```python
from build123d import *

# Parameters (mm, degrees)
F0_R     = 35
F1_DEPTH = 25
F2_R     = 50
F2_R_2   = 35
F3_DEPTH = 25


# Not quite as in the source:
# - a pattern or mirror of a feature is missing from the dataset's text; its kind, count and spacing are read off the source's solid


with BuildPart() as f1:
    # F0 (on Front) → F1 (new body, symmetric)
    with BuildSketch(Plane.XZ):
        with BuildLine():
            Line((100, 70), (-100, 70))
            ThreePointArc((-100, 70), (-170, 0), (-100, -70))
            Line((-100, -70), (100, -70))
            ThreePointArc((100, -70), (170, 0), (100, 70))
        make_face()
        with Locations((-100, 0)):
            Circle(F0_R, mode=Mode.SUBTRACT)
        with Locations((100, 0)):
            Circle(F0_R, mode=Mode.SUBTRACT)
    extrude(amount=F1_DEPTH, both=True)

    # F2 (on face) → F3 (join)
    with BuildSketch(Plane.XZ.offset(25)):
        with Locations((100, 0)):
            Circle(F2_R)
        with Locations((100, 0)):
            Circle(F2_R_2, mode=Mode.SUBTRACT)
    f3 = extrude(amount=F3_DEPTH)

    # F3_copies: F3 across plane
    add(f3.mirror(Plane.ZX))


solid = f1.part
```
Check sheet for the modelled part. Datum: model origin and axes. Units: mm. A direction names the side the tool comes from. Coordinates: 2 decimals unless noted, no trailing zeros. Write each loop counter-clockwise with the first axis right and the second up, starting at its lowest first coordinate (ties: lowest second). Pieces come first, ordered by that corner, then holes. Notation, with made-up numbers: (-27.75, 6.25) - (18.25, 6.25) arc R31 cw to (18.25, 35.25) - close; hole circle Ø3 at (66, 6.25). An arc over 180 degrees is marked (long way). One line per question, with ' | ' between items.
Item 1: Sectioned sample at B-B on y = -16.5. Record the boundary of the cut face in (x, z), plus the area to 3 significant figures.
Determined:
outline: (-100, -70) - (100, -70) arc R70 ccw to (100, 70) - (-100, 70) arc R70 ccw to start; hole circle Ø70 at (-100, 0); hole circle Ø70 at (100, 0) | area: 35,700 mm2
Item 2: Sectioned sample at A-A on z = 0. Record the boundary of the cut face in (x, y), plus the area to 3 significant figures.
Determined:
outline: (-170, -25) - (-135, -25) - (-135, 25) - (-170, 25) - close; (-65, -25) - (50, -25) - (50, -50) - (65, -50) - (65, 50) - (50, 50) - (50, 25) - (-65, 25) - close; (135, -50) - (150, -50) - (150, -25) - (170, -25) - (170, 25) - (150, 25) - (150, 50) - (135, 50) - close | area: 11,500 mm2
Item 3: Sectioned sample at C-C on y = -36.5. Record the boundary of the cut face in (x, z), plus the area to 3 significant figures.
Determined:
outline: circle Ø100 at (100, 0); hole circle Ø70 at (100, 0) | area: 4,010 mm2
Item 4: Thickness scan on line 1 (Z direction, x = -100, y = 6); line 2 (X direction, y = -3, z = 21); line 3 (Z direction, x = 100, y = -28.5). Record the ranges inside material, lowest first. Write a range as [from, to].
Determined:
line 1: z = [-70, -35], [35, 70] | line 2: x = [-166.78, -128], [-72, 72], [128, 166.78] | line 3: z = [-50, -35], [35, 50]
Item 5: Sectioned sample at D-D on z = -54. Record the boundary of the cut face in (x, y).
Determined:
outline: (-144.54, -25) - (144.54, -25) - (144.54, 25) - (-144.54, 25) - close
Item 6: Mould release check, pull along Z, two halves, no side actions. Record for faces 1 (the face through (169.983, -0.35, -1.539)), 2 (the face through (1, 0, 70)), 3 (the face through (132.33, -0.7, -13.41)): pulls with the +Z half, pulls with the -Z half, needs draft (parallel to the pull), parting line crosses it, or undercut.
Determined:
face 1: parting line crosses it | face 2: pulls with the +Z half | face 3: undercut
Item 7: Gauge pin test, flat ends, axial feed: P1, Ø1, axis at y = 17.5, z = -54.5, coming from the -X side; P2, Ø2, axis at x = 118.5, y = 5, coming from the +Z side; P3, Ø2, axis at y = 30.5, z = 10, coming from the +X side. Record the tip position at first contact, or that the pin passes through.
Determined:
P1: stops at x = -144.54 | P2: stops at z = 67.78 | P3: stops at x = 149.18
Item 8: Access from +Z, -Z, +X, -X, +Y, -Y to the whole of each face (thin tool, end or side, straight path). Record for faces 4 (the face through (50.05, -37.33, 2.2)), 5 (the face through (66, 50, -10)), 6 (the face through (50.05, 37.33, 2.2)).
Determined:
face 4: -Y | face 5: +Z, -Z, +X, -X, +Y | face 6: +Y
